Source: CAD feature listing. Evaluate the final solid. Frame: model axes, mm. Give positions to 0.01 mm unless a question says otherwise; leave off trailing zeros. Write each loop counter-clockwise with the first axis right and the second up, starting at its lowest first coordinate (ties: lowest second). Pieces come first, ordered by that corner, then holes. Notation, with made-up numbers: M -4,36 L 14,36 A23 cw 14,65 Z; hole C 85,14.5 d9. An arc over 180 degrees is marked long. Use CSV: the item, a comma, the result in double quotes. Start each with the question number.
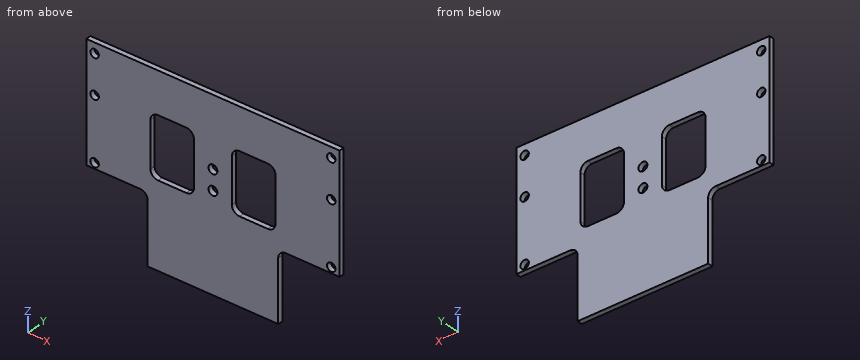
from build123d import *

# Parameters (mm, degrees)
CROQUIS1_R              = 1.65
CROQUIS1_R_2            = 1.75
SALIENTE_EXTRUIR1_DEPTH = 2


with BuildPart() as part:
    # Croquis1 → Saliente-Extruir1 (new body)
    with BuildSketch(Plane(origin=(0, 0, 0), x_dir=(1, 0, 0), z_dir=(0, 1, 0))):
        with BuildLine():
            Line((-28.5, 9.5), (-49.5, 9.5))
            Line((-49.5, 9.5), (-49.5, -36.5))
            Line((-49.5, -36.5), (49.5, -36.5))
            Line((49.5, -36.5), (49.5, 9.5))
            Line((49.5, 9.5), (28.5, 9.5))
            ThreePointArc((28.5, 9.5), (26.378679656, 10.378679656), (25.5, 12.5))
            Line((25.5, 12.5), (25.5, 36.5))
            Line((25.5, 36.5), (-25.5, 36.5))
            Line((-25.5, 36.5), (-25.5, 12.5))
            ThreePointArc((-25.5, 12.5), (-26.378679656, 10.378679656), (-28.5, 9.5))
        make_face()
        with Locations(Location((-46.25, -32.474277755, 0), (0, 0, 270))):
            Circle(CROQUIS1_R, mode=Mode.SUBTRACT)
        with Locations(Location((-46.25, -17.286108292, 0), (0, 0, 270))):
            Circle(CROQUIS1_R, mode=Mode.SUBTRACT)
        with Locations(Location((0, -9.329285485, 0), (0, 0, 270))):
            Circle(CROQUIS1_R_2, mode=Mode.SUBTRACT)
        with BuildLine():
            ThreePointArc((-10.417011027, 3.530475001), (-8.295690684, 2.651795344), (-7.417011027, 0.530475001))
            Line((-7.417011027, 0.530475001), (-7.417011027, -17.238029314))
            ThreePointArc((-7.417011027, -17.238029314), (-8.295690684, -19.359349658), (-10.417011027, -20.238029314))
            Line((-10.417011027, -20.238029314), (-21.450841414, -20.238029314))
            ThreePointArc((-21.450841414, -20.238029314), (-23.572161757, -19.359349658), (-24.450841414, -17.238029314))
            Line((-24.450841414, -17.238029314), (-24.450841414, 0.530475001))
            ThreePointArc((-24.450841414, 0.530475001), (-23.572161757, 2.651795344), (-21.450841414, 3.530475001))
            Line((-21.450841414, 3.530475001), (-10.417011027, 3.530475001))
        make_face(mode=Mode.SUBTRACT)
        with Locations(Location((0, -1.504051409, 0), (0, 0, 270))):
            Circle(CROQUIS1_R_2, mode=Mode.SUBTRACT)
        with Locations(Location((46.25, -32.474277755, 0), (0, 0, 270))):
            Circle(CROQUIS1_R, mode=Mode.SUBTRACT)
        with BuildLine():
            Line((10.417011027, 3.530475001), (21.450841414, 3.530475001))
            ThreePointArc((21.450841414, 3.530475001), (23.572161757, 2.651795344), (24.450841414, 0.530475001))
            Line((24.450841414, 0.530475001), (24.450841414, -17.238029314))
            ThreePointArc((24.450841414, -17.238029314), (23.572161757, -19.359349658), (21.450841414, -20.238029314))
            Line((21.450841414, -20.238029314), (10.417011027, -20.238029314))
            ThreePointArc((10.417011027, -20.238029314), (8.295690684, -19.359349658), (7.417011027, -17.238029314))
            Line((7.417011027, -17.238029314), (7.417011027, 0.530475001))
            ThreePointArc((7.417011027, 0.530475001), (8.295690684, 2.651795344), (10.417011027, 3.530475001))
        make_face(mode=Mode.SUBTRACT)
        with Locations(Location((46.25, -17.286108292, 0), (0, 0, 270))):
            Circle(CROQUIS1_R, mode=Mode.SUBTRACT)
        with Locations(Location((-46.25, 7.294463352, 0), (0, 0, 270))):
            Circle(CROQUIS1_R, mode=Mode.SUBTRACT)
        with Locations(Location((46.25, 7.294463352, 0), (0, 0, 270))):
            Circle(CROQUIS1_R, mode=Mode.SUBTRACT)
    extrude(amount=SALIENTE_EXTRUIR1_DEPTH)


solid = part.part
1. Section C-C on y = 1.3. Give the number of separate pieces and of enclosed holes in the cut face, then the cut area to 3 significant figures.
2. Section B-B on x = -46.25. Return loops of the section in (y, z), then the cut area to 3 significant figures.
3. Line query: probe 1 along X at (y, z) = (0.3, 12.5); probe 2 along Z at (x, y) = (19, 1.45); probe 3 along X at (y, z) = (1.25, 1). Output: solid intervals per line, ascending.
4. Section A-A on x = 15. Return loops of the section in (y, z), then the cut area to 3 significant figures.
5. Section D-D on x = 0. Return loops of the section in (y, z), then the cut area to 3 significant figures.
6. First-contact query: pin 1 (4.5 mm diameter, centred on x = 46.25, z = 17.29, fed in from +Y); pin 2 (0.6 mm diameter, centred on x = 40.5, y = 0.5, fed in from -Z); pin 3 (3 mm diameter, centred on x = -46.25, z = 17.29, fed in from +Y). Flat tips, straight axial feed; report the tip coordinate or a pass-through.
Resolved:
1,separate pieces,"1"
1,enclosed holes,"10"
1,area,"5,070 mm2"
2,outline,"M 0,-9.5 L 2,-9.5 L 2,-8.94 L 0,-8.94 Z; M 0,-5.64 L 2,-5.64 L 2,15.64 L 0,15.64 Z; M 0,18.94 L 2,18.94 L 2,30.82 L 0,30.82 Z; M 0,34.12 L 2,34.12 L 2,36.5 L 0,36.5 Z"
2,area,"72.2 mm2"
3,probe 1,"x = -49.5 to -24.45, -7.42 to 7.42, 24.45 to 49.5"
3,probe 2,"z = -36.5 to -3.53, 20.24 to 36.5"
3,probe 3,"x = -49.5 to -24.45, -7.42 to -1.68, 1.68 to 7.42, 24.45 to 49.5"
4,outline,"M 0,-36.5 L 2,-36.5 L 2,-3.53 L 0,-3.53 Z; M 0,20.24 L 2,20.24 L 2,36.5 L 0,36.5 Z"
4,area,"98.5 mm2"
5,outline,"M 0,-36.5 L 2,-36.5 L 2,-0.25 L 0,-0.25 Z; M 0,3.25 L 2,3.25 L 2,7.58 L 0,7.58 Z; M 0,11.08 L 2,11.08 L 2,36.5 L 0,36.5 Z"
5,area,"132 mm2"
6,pin 1,"stops at y = 2"
6,pin 2,"stops at z = -9.5"
6,pin 3,"passes through"
